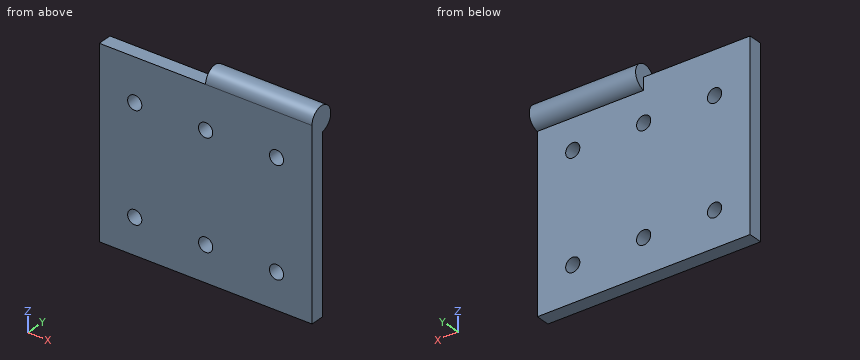
from build123d import *

# Parameters (mm, degrees)
SKETCH1_W           = 15
SKETCH1_H           = 13
BOSS_EXTRUDE1_DEPTH = 1
SKETCH2_R           = 0.875
BOSS_EXTRUDE2_DEPTH = 7.5
SKETCH3_R           = 0.5
CUT_EXTRUDE1_DEPTH  = 2


with BuildPart() as part:
    # Sketch1 → Boss-Extrude1 (new body)
    with BuildSketch(Plane(origin=(0, 0, 0), x_dir=(1, 0, 0), z_dir=(0, 1, 0))):
        with Locations((10.569631841, -166.54341444)):
            Rectangle(SKETCH1_W, SKETCH1_H)
    extrude(amount=BOSS_EXTRUDE1_DEPTH)

    # Sketch2 → Boss-Extrude2 (add)
    with BuildSketch(Plane(origin=(18.069631841, 0, 0), x_dir=(0, 0, -1), z_dir=(1, 0, 0))):
        with Locations((-173.04341444, 0.875)):
            Circle(SKETCH2_R)
    extrude(amount=-BOSS_EXTRUDE2_DEPTH)

    # Sketch3 → Cut-Extrude1 (cut, through all)
    with BuildSketch(Plane(origin=(0, 1, 0), x_dir=(1, 0, 0), z_dir=(0, 1, 0))):
        with Locations((15.569631841, -162.54341444)):
            Circle(SKETCH3_R)
        with Locations((15.569631841, -170.04341444)):
            Circle(SKETCH3_R)
        with Locations((10.569631841, -162.54341444)):
            Circle(SKETCH3_R)
        with Locations((10.569631841, -170.04341444)):
            Circle(SKETCH3_R)
        with Locations((5.569631841, -162.54341444)):
            Circle(SKETCH3_R)
        with Locations((5.569631841, -170.04341444)):
            Circle(SKETCH3_R)
    extrude(amount=-CUT_EXTRUDE1_DEPTH, mode=Mode.SUBTRACT)


solid = part.part
Read the model definition and answer for the solid it produces. Units are mm, in the model's axes. Give positions to 0.01 mm unless a question says otherwise; leave off trailing zeros. Loops run counter-clockwise (first coordinate to the right, second up) from the corner with the lowest first, then second, coordinate; pieces in that order, holes last. Notation, with made-up numbers: (-20.5, 84) -> (-7.5, 84) arc R21 cw to (-7.5, 110) -> close; hole circle Ø2 at (87.25, 82). An arc over 180 degrees is marked (long way). Use a Markdown table: item, result.
Q1. Find the intervals of material crossed by line 1 along Z through (x, y) = (16, 0.8); line 2 along X through (y, z) = (0.6, 169.75); line 3 along Z through (x, y) = (9.75, 0.9), in increasing order.
Solved:
| item | result |
|---|---|
| line 1 | z = 160.04 to 162.29, 162.8 to 169.79, 170.3 to 173.92 |
| line 2 | x = 3.07 to 5.16, 5.97 to 10.16, 10.97 to 15.16, 15.97 to 18.07 |
| line 3 | z = 160.04 to 173.04 |
Q2. Section B-B, the plane x = 9 is taken. Determine the outline of the cut face in (y, z), then the cut area to 3 significant figures.
Solved:
| item | result |
|---|---|
| outline | (0, 160.04) -> (1, 160.04) -> (1, 173.04) -> (0, 173.04) -> close |
| area | 13.0 mm^2 |
Q3. Section A-A, the plane z = 167.5 is taken. Determine the outline of the cut face in (x, y).
Solved:
| item | result |
|---|---|
| outline | (3.07, 0) -> (18.07, 0) -> (18.07, 1) -> (3.07, 1) -> close |
